Autodesk Inventor part; units mm, degrees
ref_plane "YZ Plane" through (0, 0, 0) normal (1, 0, 0) x (0, 1, 0)
ref_plane "XZ Plane" through (0, 0, 0) normal (0, 1, 0) x (-1, 0, 0)
ref_plane "XY Plane" through (0, 0, 0) normal (0, 0, 1) x (1, 0, 0)
sketch "Sketch1" plane through (0, 0, 0) normal (0, 1, 0) x (-1, 0, 0)
  line L0 (0, 0) -> (69, 0)
  line L1 (69, 0) -> (69, -41)
  line L2 (69, -41) -> (0, -41)
  line L3 (0, -41) -> (0, 0)
  line L4 (-3, 3) -> (72, 3)
  line L5 (72, 3) -> (72, -44)
  line L6 (72, -44) -> (-3, -44)
  line L7 (-3, -44) -> (-3, 3)
  dimension "d0" = 69
  dimension "d1" = 41
  dimension "d2" = 3
extrude "Extrusion1" add sketch "Sketch1" along normal blind 18.5
sketch "Sketch2" plane through (0, 18.5, 0) normal (0, 1, 0) x (1, 0, 0)
  line L0 (0, 0) -> (-69, 0)
  line L1 (-69, 41) -> (0, 41)
  line L2 (-69, 0) -> (0, 0)
  line L3 (0, 0) -> (0, 41)
  line L4 (0, 41) -> (-69, 41)
  line L5 (-69, 41) -> (-69, 0)
  line L6 (0.2, 41.2) -> (0.2, -0.2)
  line L7 (0.2, -0.2) -> (-69.2, -0.2)
  line L8 (-69.2, -0.2) -> (-69.2, 41.2)
  line L9 (-69.2, 41.2) -> (0.2, 41.2)
  dimension "d5" = 0.2
extrude "Extrusion2" cut sketch "Sketch2" against normal blind 18.5
sketch "Sketch3" plane through (0, 18.5, 0) normal (0, 1, 0) x (1, 0, 0)
  line L0 (-72, -3) -> (3, -3)
  line L1 (3, -3) -> (3, 44)
  line L2 (-72, -3) -> (3, -3)
  line L3 (3, -3) -> (3, 44)
  line L4 (3, 44) -> (-72, 44)
  line L5 (-72, 44) -> (-72, -3)
  point P0 (0, 0)
extrude "Extrusion3" add sketch "Sketch3" along normal blind 1
sketch "Sketch4" plane through (0, 19.5, 0) normal (0, 1, 0) x (1, 0, 0)
  line L0 (3, -3) -> (3, 44)
  line L1 (3, 44) -> (-72, 44)
  line L2 (3, -3) -> (-72, 44)
  circle A0 centre (-34.5, 20.5) radius 5
  point P0 (0, 0)
  dimension "d10" = 10
extrude "Extrusion4" cut sketch "Sketch4" against normal blind 1 contours A0 L2 | L2 A0
properties part number "top batt cage"
CAD build for the part. Positions are in the model's coordinates, mm. A direction names the side the tool comes from. Coordinates: 2 decimals unless noted, no trailing zeros. Loops run counter-clockwise (first coordinate to the right, second up) from the corner with the lowest first, then second, coordinate; pieces in that order, holes last. Notation, with made-up numbers: (-18.5, 42) - (28.5, 42) arc R8 ccw to (28.5, 50) - close; hole circle Ø8 at (-30.5, 89.5). An arc over 180 degrees is marked (long way). Use CSV: the item, a comma, the result in double quotes. Start each with the question number.
Q1. Cut at B-B, the plane z = -20.5. List the corners of the cut face in (x, y), then the cut area to 3 significant figures.
Q2. Cut at A-A, the plane x = -34.5. List the corners of the cut face in (y, z).
Q3. Drop flat-ended pins along their axis: P1, Ø8, axis at x = -34.5, z = -20.5, coming from the -Y side; P2, Ø10, axis at x = -35.5, z = -25, coming from the -Y side. Give the stop position or say it passes through.
Q4. Probe probe 1 along X at (y, z) = (2.5, -27.5); probe 2 along X at (y, z) = (19.15, -20.5); probe 3 along Z at (x, y) = (-53, 13.5). List the from-to ranges inside material, lowest first. Write a range as from..to.
Q5. 3-axis set-ups, long thin cutter, end or side, ignore diameter. For faces 1 (the flat face through (-35, 9, -41.2)), 2 (the flat face through (-35, 10, 3)): which of +Z, -Z, +X, -X, +Y, -Y reach the whole face in a straight line?
Q6. Two-plate mould, pull along X, no slides. Class faces 3 (the flat face through (0.2, 9, -21)), 4 (the flat face through (-34, 10, -44)), 5 (the flat face through (-72, 10, -21)): +X half, -X half, draft (parallel to the pull), parting line (faces both ways), or undercut.
Q7. Cut at D-D, the plane x = -1.5. List the corners of the cut face in (y, z), then the cut area to 3 significant figures.
Q8. Cut at C-C, the plane y = 15.75. List the corners of the cut face in (x, z).
Here are the results:
1,outline,"(-72, 0) - (-69.2, 0) - (-69.2, 18.5) - (-39.5, 18.5) - (-39.5, 19.5) - (-72, 19.5) - close; (-29.5, 18.5) - (0.2, 18.5) - (0.2, 0) - (3, 0) - (3, 19.5) - (-29.5, 19.5) - close"
1,area,"169 mm2"
2,outline,"(0, -44) - (19.5, -44) - (19.5, -25.5) - (18.5, -25.5) - (18.5, -41.2) - (0, -41.2) - close; (0, 0.2) - (18.5, 0.2) - (18.5, -15.5) - (19.5, -15.5) - (19.5, 3) - (0, 3) - close"
3,P1,"through"
3,P2,"y = 18.5"
4,probe 1,"-72..-69.2, 0.2..3"
4,probe 2,"-72..-39.5, -29.5..3"
4,probe 3,"-44..-41.2, 0.2..3"
5,face 1,"-Y"
5,face 2,"+Z, +X, -X, +Y, -Y"
6,face 3,"undercut"
6,face 4,"draft"
6,face 5,"-X half"
7,outline,"(0, -44) - (19.5, -44) - (19.5, 3) - (0, 3) - (0, 0.2) - (18.5, 0.2) - (18.5, -41.2) - (0, -41.2) - close"
7,area,"151 mm2"
8,outline,"(-72, -44) - (3, -44) - (3, 3) - (-72, 3) - close; hole (-69.2, -41.2) - (0.2, -41.2) - (0.2, 0.2) - (-69.2, 0.2) - close"
